from build123d import *

# Parameters (mm, degrees)
SKETCH4_W                 = 2.05
SKETCH4_H                 = 0.8
SKETCH5_OUTSIDE_W         = 11.37
SKETCH5_OUTSIDE_H         = 11.37
CUT_INNER_BODY_DEPTH      = 1.5
CUT_INNER_BODY_DEPTH_BACK = 1.3
FILLET_2_R                = 0.3


with BuildPart() as part:
    # Sketch4 → Clip (revolve)
    with BuildSketch(Plane.XY):
        with Locations((2.625, 0.1)):
            Rectangle(SKETCH4_W, SKETCH4_H)
    revolve(axis=Axis((0, 0.5, 0), (0, -1, 0)))

    # Sketch5 outside → Cut-Inner-Body (cut, two sides)
    with BuildSketch(Plane(origin=(0, 0, 0), x_dir=(1, 0, 0), z_dir=(0, 1, 0))) as cut_inner_body_sk:
        Rectangle(SKETCH5_OUTSIDE_W, SKETCH5_OUTSIDE_H)
        with BuildLine():
            Line((2.566160275, -2.595635075), (1.35, -0.858778202))
            ThreePointArc((1.35, -0.858778202), (1.569360567, -0.31162062), (1.575692405, 0.277837084))
            Line((1.575692405, 0.277837084), (2.585120352, 0.455826466))
            ThreePointArc((2.585120352, 0.455826466), (2.150274116, 1.505638145), (1.3125, 2.273316685))
            Line((1.3125, 2.273316685), (0.8, 1.385640646))
            ThreePointArc((0.8, 1.385640646), (0, 1.6), (-0.8, 1.385640646))
            Line((-0.8, 1.385640646), (-1.3125, 2.273316685))
            ThreePointArc((-1.3125, 2.273316685), (-2.150274116, 1.505638145), (-2.585120352, 0.455826466))
            Line((-2.585120352, 0.455826466), (-1.575692405, 0.277837084))
            ThreePointArc((-1.575692405, 0.277837084), (-1.569360567, -0.31162062), (-1.35, -0.858778202))
            Line((-1.35, -0.858778202), (-2.566160275, -2.595635075))
            ThreePointArc((-2.566160275, -2.595635075), (0, 3.65), (2.566160275, -2.595635075))
        make_face(mode=Mode.SUBTRACT)
    extrude(amount=CUT_INNER_BODY_DEPTH, mode=Mode.SUBTRACT)
    extrude(cut_inner_body_sk.sketch, amount=-CUT_INNER_BODY_DEPTH_BACK, mode=Mode.SUBTRACT)

    # Fillet 2
    fillet_2_edges = [part.edges().sort_by_distance(p)[0] for p in [
        (2.566160275, 0.1, 2.595635075),
        (1.35, 0.1, 0.858778202),
        (1.575692405, 0.1, -0.277837084),
        (2.585120352, 0.1, -0.455826466),
        (1.3125, 0.1, -2.273316685),
        (0.8, 0.1, -1.385640646),
        (-0.8, 0.1, -1.385640646),
        (-1.3125, 0.1, -2.273316685),
        (-2.585120352, 0.1, -0.455826466),
        (-1.575692405, 0.1, -0.277837084),
        (-1.35, 0.1, 0.858778202),
        (-2.566160275, 0.1, 2.595635075),
    ]]
    fillet(fillet_2_edges, radius=FILLET_2_R)


solid = part.part
Model file for the job. Use its own axes, mm. A direction names the side the tool comes from. Give positions to 0.01 mm unless a question says otherwise; leave off trailing zeros. Order: outer loops, then holes, each group sorted by start corner. A loop starts at its lowest first (then second) coordinate and runs counter-clockwise, first axis right, second up. Notation, with made-up numbers: M 85,36 L 133,36 A21 ccw 133,53 Z; hole C 76,5 d1. An arc over 180 degrees is marked long. Put each result on its own line as item: value. Start each with the question number.
(1) Pin check, flat tip, straight feed: pin 1 Ø1.5 at (x, z) = (-0.5, -0.5) entering from +Y. Stop position of the tip, or through.
(2) Band-saw the part on C-C on z = -3. Give the cut face in (x, y).
(3) Drill centre lines: L1, parallel to X at y = 0.45, z = 1.25; L2, parallel to X at y = 0.45, z = -2; L3, parallel to X at y = -0.1, z = -1.25. Where is each one in solid material? Low to high. Write a range as [from, to].
(4) Pull direction Z, two halves, no side cores. Call faces 4 (the face through (-0.12, 0.11, -3.65)), 5 (the face through (2.157, 0.106, -1.496)), 6 (the face through (1.91, 0.11, 1.66)), 7 (the face through (0, -0.3, -2)): released by +Z, released by -Z, zero draft, split by the parting line, or undercut.
(5) Band-saw the part on A-A on x = 0. Give the cut face in (y, z).
(6) Tool access for faces 1 (the face through (0, 0.5, -2)), 2 (the face through (-1.898, 0.106, 1.642)), 3 (the face through (-2.144, 0.106, -1.515)): list every direction of +Z, -Z, +X, -X, +Y, -Y with a clear straight run to the whole face (end or side of a thin tool).
(7) Band-saw the part on B-B on y = 0.15. Give the cut face in (x, z) (3 decimals), then the cut area to 3 significant figures.
Results below:
1. pin 1: passes through
2. outline: M -2.08,-0.3 L 2.08,-0.3 L 2.08,0.5 L -2.08,0.5 Z
3. L1: x = [-3.43, -1.62], [1.62, 3.43]
3. L2: x = [-3.05, -1.7], [-1.15, 1.15], [1.7, 3.05]
3. L3: x = [-3.43, -2.31], [2.31, 3.43]
4. face 4: split by the parting line
4. face 5: undercut
4. face 6: released by +Z
4. face 7: zero draft
5. outline: M -0.3,-3.65 L 0.5,-3.65 L 0.5,-1.6 L -0.3,-1.6 Z
6. face 1: +Z, -Z, +X, -X, +Y
6. face 2: +Z, +Y, -Y
6. face 3: +Y, -Y
7. outline: M -2.829,2.306 A3.65 ccw long 2.829,2.306 A0.3 ccw 2.351,2.288 L 1.458,1.013 A0.3 ccw 1.435,0.708 A1.6 cw 1.6,-0.026 A0.3 ccw 1.848,-0.326 L 2.271,-0.4 A0.3 cw 2.505,-0.786 A2.625 cw 1.595,-2.085 A0.3 cw 1.153,-1.997 L 0.938,-1.625 A0.3 ccw 0.571,-1.495 A1.6 cw -0.571,-1.495 A0.3 ccw -0.938,-1.625 L -1.153,-1.997 A0.3 cw -1.595,-2.085 A2.625 cw -2.505,-0.786 A0.3 cw -2.271,-0.4 L -1.848,-0.326 A0.3 ccw -1.6,-0.026 A1.6 cw -1.435,0.708 A0.3 ccw -1.458,1.013 L -2.351,2.288 A0.3 ccw Z
7. area: 20.9 mm2
